Geometry: see drawing. Coordinates: mm, zero at the bounding-box minimum. A direction names the side the tool comes from. Round coordinates to 2 decimals unless told otherwise and drop trailing zeros. Order: outer loops, then holes, each group sorted by start corner. A loop starts at its lowest first (then second) coordinate and runs counter-clockwise, first axis right, second up. Notation, with made-up numbers: (26, 71.5) - (79, 71.5) arc R9 cw to (79, 81.5) - close; hole circle Ø11 at (18.25, 23.5). An arc over 180 degrees is marked (long way). Put each result on its own line as item: value. Start each with the question number.
1) Section B-B on z = 16.5. Output: boundary loops of the cut face in (x, y), then the cut area to 3 significant figures.
2) Line query: probe 1 along Y at (x, z) = (10, 6.65); probe 2 along Y at (x, z) = (10, 1.9); probe 3 along Z at (x, y) = (7.5, 46.5). Output: solid intervals per line, ascending. Write a range as [from, to].
3) Section D-D on y = 59.5. Output: boundary loops of the cut face in (x, z).
4) Section A-A on y = 50. Output: boundary loops of the cut face in (x, z), then the cut area to 4 significant figures.
5) Section C-C on z = 4. Output: boundary loops of the cut face in (x, y).
6) Contact query for flat-ended pins moving along their axis: P1, Ø9, axis at x = 10, y = 30, coming from the +Z side; P2, Ø3.5, axis at x = 8, y = 67.5, coming from the -Z side; P3, Ø4, axis at y = 45.5, z = 29, coming from the -X side. Output: stop coordinate, or through.
7) Access query for the marked faces 1 and 2. Directions: +Z, -Z, +X, -X, +Y, -Y. A direction counts if a zero-diameter tool reaches every point of the face in a straight line with its end or side. Return the directions, or none.
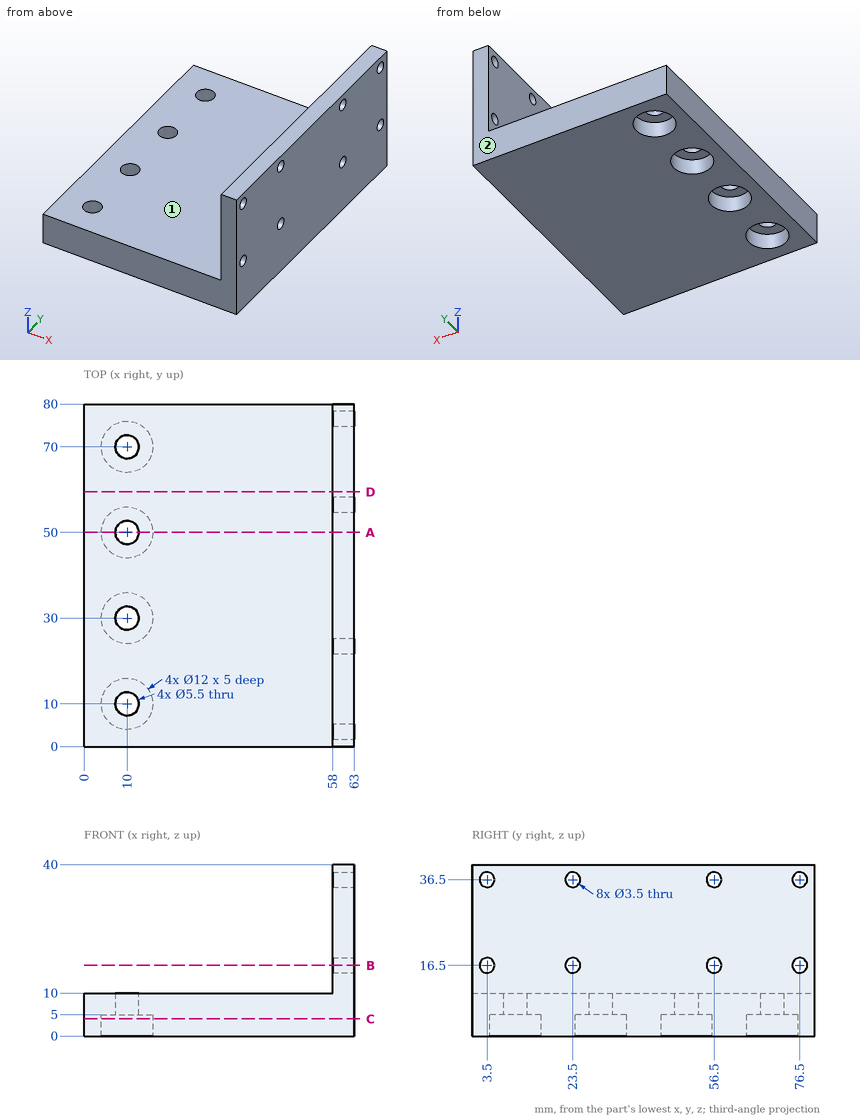
Answer sheet:
1. outline: (58, 0) - (63, 0) - (63, 1.75) - (58, 1.75) - close; (58, 5.25) - (63, 5.25) - (63, 21.75) - (58, 21.75) - close; (58, 25.25) - (63, 25.25) - (63, 54.75) - (58, 54.75) - close; (58, 58.25) - (63, 58.25) - (63, 74.75) - (58, 74.75) - close; (58, 78.25) - (63, 78.25) - (63, 80) - (58, 80) - close
1. area: 330 mm^2
2. probe 1: [0, 7.25], [12.75, 27.25], [32.75, 47.25], [52.75, 67.25], [72.75, 80]
2. probe 2: [0, 4], [16, 24], [36, 44], [56, 64], [76, 80]
2. probe 3: [5, 10]
3. outline: (0, 0) - (63, 0) - (63, 40) - (58, 40) - (58, 10) - (0, 10) - close
4. outline: (0, 0) - (4, 0) - (4, 5) - (7.25, 5) - (7.25, 10) - (0, 10) - close; (12.75, 5) - (16, 5) - (16, 0) - (63, 0) - (63, 40) - (58, 40) - (58, 10) - (12.75, 10) - close
4. area: 692.5 mm^2
5. outline: (0, 0) - (63, 0) - (63, 80) - (0, 80) - close; hole circle Ø12 at (10, 10); hole circle Ø12 at (10, 30); hole circle Ø12 at (10, 50); hole circle Ø12 at (10, 70)
6. P1: z = 10
6. P2: z = 5
6. P3: x = 58
7. face 1: +Z, -X, +Y, -Y
7. face 2: +Z, -Z, +X, -X, +Y
